Could you check a few things on this model? Use its own coordinates, in mm. A direction names the side the tool comes from. Give positions to 0.01 mm unless a question says otherwise; leave off trailing zeros. Write each loop counter-clockwise with the first axis right and the second up, starting at its lowest first coordinate (ties: lowest second). Pieces come first, ordered by that corner, then holes. Notation, with made-up numbers: (77.25, 15.25) - (103.25, 15.25) arc R18 cw to (103.25, 43.25) - close; hole circle Ø9 at (78.5, 77). An arc over 180 degrees is marked (long way). Answer as CSV lines item,"result". Start each with the question number.
Q1. If I drill on line 1 along Z through (x, y) = (35, 24.5); line 2 along Y through (x, z) = (42, -54); line 3 along Z through (x, y) = (63, 24), over which ranges is the centre line in solid material (lowest first)?
Q2. Imagine slicing it at D-D on z = -40.5. List the corners of the cut face in (x, y) for me, and give its area (3 significant figures).
Q3. Imagine slicing it at C-C on z = 8. List the corners of the cut face in (x, y) for me.
Q4. Will these pins go through, and if not, where does the flat tip stop? pin 1 Ø1.5 at (x, y) = (65, -12.5) entering from -Z; pin 2 Ø1.3 at (x, z) = (6.5, -1.5) entering from -Y; pin 3 Ø12 at (x, z) = (28, -12) entering from -Y.
Q5. Imagine slicing it at A-A on x = 35. List the corners of the cut face in (y, z) for me, and give its area (3 significant figures).
Q6. On a 3-axis mill with a long thin cutter (end or side, diameter ignored), from which of +Z, -Z, +X, -X, +Y, -Y can I reach the whole of each face in a straight line? I mean faces 1 (the face through (37.168, 23.042, -44.505)), 2 (the face through (5, -12, 0)). Say none if no direction works.
Q7. We'd pull the mould along X, two halves only. Please class faces 3 (the face through (70, 12, -6)), 4 (the face through (10.2, 23, -33.3)), 5 (the face through (5, 9.75, -1)): pulls with the +X half, pulls with the -X half, needs draft (parallel to the pull), parting line crosses it, or undercut.
Q8. Imagine slicing it at B-B on y = 0. List the corners of the cut face in (x, z) for me.
```python
from build123d import *

# Parameters (mm, degrees)
F1_DEPTH  = 70
F4_W      = 50
F4_H      = 24.5480843189
F5_DEPTH  = 25
F7_DEPTH  = 40.7510000745
F8_R      = 10
F9_DEPTH  = 40.7510000745
F10_R     = 6.38
F11_DEPTH = 40.7510000745
F6_R      = 4
F12_DEPTH = 40.7510000745
F15_DEPTH = 10
F16_R     = 4
F17_DEPTH = 40.7510000745
F19_DEPTH = 10


# Not quite as in the source:
# - a pattern or mirror of a feature is missing from the dataset's text; its kind, count and spacing are read off the source's solid


with BuildPart() as f1:
    # F0 (on Right) → F1 (new body)
    with BuildSketch(Plane.YZ):
        with BuildLine():
            ThreePointArc((-9.75, 0), (0, 9.75), (9.75, 0))
            Line((9.75, 0), (9.75, -2.5980842444))
            Line((9.75, -2.5980842444), (20, -9.7980842444))
            Line((20, -9.7980842444), (20, -69.7980842444))
            Line((20, -69.7980842444), (26, -69.7980842444))
            Line((26, -69.7980842444), (26, -7.9024389721))
            Line((26, -7.9024389721), (14.7500000745, 0))
            ThreePointArc((14.7500000745, 0), (0, 14.7500000745), (-14.7500000745, 0))
            Line((-14.7500000745, 0), (-9.75, 0))
        make_face()
    extrude(amount=F1_DEPTH)

    # F4 (on face) → F5 (cut)
    with BuildSketch(Plane(origin=(0, 26, 0), x_dir=(-1, 0, 0), z_dir=(0, 1, 0))):
        Polygon((-45, -69.7980842444), (-70, -34.7980842444), (-90, -34.7980842444), (-90, -94.7980842444), (20, -94.7980842444), (20, -34.7980842444), (0, -34.7980842444), (-25, -69.7980842444), align=None)
        with Locations((-35, 2.475957915)):
            Rectangle(F4_W, F4_H)
    extrude(amount=-F5_DEPTH, mode=Mode.SUBTRACT)

    # F4 (on face) → F7 (cut, through all)
    with BuildSketch(Plane(origin=(0, 26, 0), x_dir=(-1, 0, 0), z_dir=(0, 1, 0))):
        Polygon((-45, -69.7980842444), (-70, -34.7980842444), (-90, -34.7980842444), (-90, -94.7980842444), (20, -94.7980842444), (20, -34.7980842444), (0, -34.7980842444), (-25, -69.7980842444), align=None)
        with Locations((-35, 2.475957915)):
            Rectangle(F4_W, F4_H)
    extrude(amount=-F7_DEPTH, mode=Mode.SUBTRACT)

    # F8 (on face) → F9 (cut, through all)
    with BuildSketch(Plane(origin=(0, 26, 0), x_dir=(-1, 0, 0), z_dir=(0, 1, 0))):
        with Locations((-35, -34.7424389721)):
            Circle(F8_R)
    extrude(amount=-F9_DEPTH, mode=Mode.SUBTRACT)

    # F10 (on face) → F11 (cut, through all)
    with BuildSketch(Plane(origin=(0, 26, 0), x_dir=(-1, 0, 0), z_dir=(0, 1, 0))):
        with Locations((-35, -34.7424389721)):
            Circle(F10_R)
    extrude(amount=-F11_DEPTH, mode=Mode.SUBTRACT)

    # F6 (on face) → F12 (cut, through all)
    with BuildSketch(Plane(origin=(0, 26, 0), x_dir=(-1, 0, 0), z_dir=(0, 1, 0))):
        with Locations((-63, -30.9024389721)):
            Circle(F6_R)
        with Locations((-7, -30.9024389721)):
            Circle(F6_R)
    extrude(amount=-F12_DEPTH, mode=Mode.SUBTRACT)

    # F14 (on face) → F15 (join)
    with BuildSketch(Plane(origin=(0, 0, 0), x_dir=(0, -1, 0), z_dir=(-1, 0, 0))):
        Polygon((-20, -9.7980842444), (-20, -25.9981378913), (-9.75, -2.5980842444), align=None)
    f15 = extrude(amount=-F15_DEPTH)

    # F15_copies: F15 across plane
    add(f15.mirror(Plane(origin=(35, 0, 0), x_dir=(0, 0, 1), z_dir=(1, 0, 0))))

    # F16 (on face) → F17 (cut, through all)
    with BuildSketch(Plane(origin=(0, 26, 0), x_dir=(-1, 0, 0), z_dir=(0, 1, 0))):
        with Locations((-35, -61.7980842444)):
            Circle(F16_R)
    extrude(amount=-F17_DEPTH, mode=Mode.SUBTRACT)

    # F18 (on face) → F19 (join)
    with BuildSketch(Plane(origin=(0, 0, 0), x_dir=(0, -1, 0), z_dir=(-1, 0, 0))):
        Polygon((-11.2626504483, 9.5244531117), (-26, -7.9024389721), (-14.7500000745, 0), align=None)
    f19 = extrude(amount=-F19_DEPTH)

    # F19_copies: F19 across plane
    add(f19.mirror(Plane(origin=(35, 0, 0), x_dir=(0, 0, 1), z_dir=(1, 0, 0))))


solid = f1.part
```
Conclusion:
1,line 1,"-69.8 to -65.8, -57.8 to -44.74, -24.74 to -9.8"
1,line 2,"20 to 26"
1,line 3,"-44.6 to -34.9, -26.9 to -5.54"
2,outline,"(4.07, 20) - (26.82, 20) - (26.82, 26) - (4.07, 26) - close; (43.18, 20) - (65.93, 20) - (65.93, 26) - (43.18, 26) - close"
2,area,"273 mm^2"
3,outline,"(0, -12.39) - (10, -12.39) - (10, -5.57) - (0, -5.57) - close; (0, 5.57) - (10, 5.57) - (10, 12.55) - (0, 12.55) - close; (60, -12.39) - (70, -12.39) - (70, -5.57) - (60, -5.57) - close; (60, 5.57) - (70, 5.57) - (70, 12.55) - (60, 12.55) - close"
4,pin 1,"z = 0"
4,pin 2,"y = 9.75"
4,pin 3,"y = 20"
5,outline,"(20, -69.8) - (26, -69.8) - (26, -65.8) - (20, -65.8) - close; (20, -57.8) - (26, -57.8) - (26, -44.74) - (20, -44.74) - close; (20, -24.74) - (26, -24.74) - (26, -9.8) - (20, -9.8) - close"
5,area,"192 mm^2"
6,face 1,"+Y, -Y"
6,face 2,"-Z, +X, -X, -Y"
7,face 3,"pulls with the +X half"
7,face 4,"undercut"
7,face 5,"needs draft"
8,outline,"(0, 9.75) - (10, 9.75) - (10, 14.75) - (0, 14.75) - close; (60, 9.75) - (70, 9.75) - (70, 14.75) - (60, 14.75) - close"
